```python
from build123d import *

# Parameters (mm, degrees)
F0_R          = 17.5
F1_DEPTH      = 600
F2_R          = 11.5
F3_DEPTH      = 77.4004622785
F3_DEPTH_BACK = 26.2177260049
F5_W          = 169
F5_H          = 33.3154127554
F6_DEPTH      = 50
F7_R          = 15
F8_DEPTH      = 25


with BuildPart() as f1:
    # F0 (on Top) → F1 (new body)
    with BuildSketch(Plane.XY):
        with Locations((-39.4086318632, 0)):
            Circle(F0_R)
    extrude(amount=F1_DEPTH)



with BuildPart() as f1b:
    # F0 (on Top) → F1, piece 2 (new body)
    with BuildSketch(Plane.XY):
        with Locations((90.5913681368, 0)):
            Circle(F0_R)
    extrude(amount=F1_DEPTH)


with BuildPart() as f1_1:
    add(f1.part)

    add(f1b.part)  # F3 merges F1b
    # F2 (on Right) → F3 (join, two sides)
    with BuildSketch(Plane.YZ) as f3_sk:
        with Locations((0, 34.3021339912)):
            Circle(F2_R)
    extrude(amount=F3_DEPTH)
    extrude(f3_sk.sketch, amount=-F3_DEPTH_BACK)

    # F5 (on offset) → F6 (join)
    with BuildSketch(Plane.XY.offset(630)):
        with Locations((24.0950547159, 0.109818764)):
            Rectangle(F5_W, F5_H)
    extrude(amount=-F6_DEPTH)

    # F7 (on face) → F8 (join)
    with BuildSketch(Plane.XY.offset(630)):
        with Locations((24.0950547159, 0)):
            Circle(F7_R)
    extrude(amount=F8_DEPTH)


solid = f1_1.part
```
CAD build for the part. Positions are in the model's coordinates, mm. A direction names the side the tool comes from. Round coordinates to 2 decimals unless told otherwise and drop trailing zeros. Order: outer loops, then holes, each group sorted by start corner. A loop starts at its lowest first (then second) coordinate and runs counter-clockwise, first axis right, second up. Notation, with made-up numbers: (58, 39) - (101, 39) arc R19 cw to (101, 55) - close; hole circle Ø6 at (-13, 48.25). An arc over 180 degrees is marked (long way). Answer as CSV lines item,"result". Start each with the question number.
1. Pin check, flat tips, straight feed: pin 1 (10 mm diameter, centred on x = 57, y = 0, fed in from -Z); pin 2 (5 mm diameter, centred on x = -16, y = 12, fed in from -Z); pin 3 (1 mm diameter, centred on x = -38, y = -17, fed in from +Z). Stop position of each tip, or through.
2. Pull direction Z, two halves, no side cores. Call faces 6 (the face through (108.595, 0, 605)), 7 (the face through (25, 0, 580)), 8 (the face through (90, 0, 0)), 9 (the face through (26.317, -2.493, 23.076)): +Z half, -Z half, draft (parallel to the pull), parting line (faces both ways), or undercut.
3. Saw through at C-C, the plane z = 220. Write the cut outline in (x, y), and give its area (3 significant figures).
4. Tool access for faces 1 (the face through (106.76, -6.7, 295.8)), 2 (the face through (-58, 0, 580)), 3 (the face through (-40, 0, 0)), 4 (the face through (38.4, 4.51, 642.33)), 5 (the face through (108.3, 1.4, 580)): list every direction of +Z, -Z, +X, -X, +Y, -Y with a clear straight run to the whole face (end or side of a thin tool).
5. Saw through at B-B, the plane x = -10.5. Write the cut outline in (y, z).
6. Saw through at A-A, the plane y = 0. Write the cut outline in (x, z), and give its area (3 significant figures).
7. Drill centre lines: L1, parallel to X at y = -2, z = 401.5; L2, parallel to X at y = 0.5, z = 540; L3, parallel to Z at x = 45, y = 0. Where is each one in solid material? Low to high. Write a range as [from, to].
Model answer:
1,pin 1,"stops at z = 22.8"
1,pin 2,"stops at z = 27.82"
1,pin 3,"stops at z = 630"
2,face 6,"draft"
2,face 7,"undercut"
2,face 8,"-Z half"
2,face 9,"undercut"
3,outline,"circle Ø35 at (-39.41, 0); circle Ø35 at (90.59, 0)"
3,area,"1,920 mm²"
4,face 1,"none"
4,face 2,"-Z, -X"
4,face 3,"-Z, +X, -X, +Y, -Y"
4,face 4,"+Z"
4,face 5,"-Z, +X"
5,outline,"(-16.55, 580) - (16.77, 580) - (16.77, 630) - (-16.55, 630) - close; circle Ø23 at (0, 34.3)"
6,outline,"(-60.4, 580) - (-56.91, 580) - (-56.91, 0) - (-21.91, 0) - (-21.91, 22.8) - (73.09, 22.8) - (73.09, 0) - (108.09, 0) - (108.09, 580) - (108.6, 580) - (108.6, 630) - (39.1, 630) - (39.1, 655) - (9.1, 655) - (9.1, 630) - (-60.4, 630) - close; hole (-21.91, 45.8) - (73.09, 45.8) - (73.09, 580) - (-21.91, 580) - close"
6,area,"52,000 mm²"
7,L1,"x = [-56.79, -22.02], [73.21, 107.98]"
7,L2,"x = [-56.9, -21.92], [73.1, 108.08]"
7,L3,"z = [22.8, 45.8], [580, 630]"
